Geometry check sheet. Reference: the model listing, model coordinates, mm. A direction names the side the tool comes from. Give positions to 0.01 mm unless a question says otherwise; leave off trailing zeros. Order: outer loops, then holes, each group sorted by start corner. A loop starts at its lowest first (then second) coordinate and runs counter-clockwise, first axis right, second up.
from build123d import *

# Parameters (mm, degrees)
SKETCH1_W           = 75
SKETCH1_H           = 15
BOSS_EXTRUDE1_DEPTH = 15
BOSS_EXTRUDE2_DEPTH = 7.5


with BuildPart() as part:
    # Sketch1 → Boss-Extrude1 (new, symmetric)
    with BuildSketch(Plane(origin=(0, 0, 0), x_dir=(-1, 0, 0), z_dir=(0, 1, 0))):
        with Locations((0, 7.5)):
            Rectangle(SKETCH1_W, SKETCH1_H)
    extrude(amount=BOSS_EXTRUDE1_DEPTH, both=True)

    # Sketch1_3 → Boss-Extrude2 (add, symmetric)
    with BuildSketch(Plane(origin=(0, 0, 0), x_dir=(-1, 0, 0), z_dir=(0, 1, 0))):
        Polygon((-22.5, 90), (-22.5, 15), (22.5, 15), (22.5, 90), (0, 112.5), align=None)
    extrude(amount=BOSS_EXTRUDE2_DEPTH, both=True)


solid = part.part
Item 1: Set-up check for faces 1 (the flat face through (0, -7.5, 64)), 2 (the flat face through (0, 7.5, 64)), 3 (the flat face through (-22.5, 0, 52)), 4 (the flat face through (22.5, 0, 53)), 5 (the flat face through (1, 0, 0)): record each of +Z, -Z, +X, -X, +Y, -Y from which the full face is reachable in a straight line by a thin tool's end or side.
Reported:
face 1: +Z, +X, -X, -Y
face 2: +Z, +X, -X, +Y
face 3: +Z, -X, +Y, -Y
face 4: +Z, +X, +Y, -Y
face 5: -Z, +X, -X, +Y, -Y
Item 2: Sectioned sample at B-B (y = -4.25). Enter the section's corners in (x, z).
Reported:
outline: (-37.5, 0) - (37.5, 0) - (37.5, 15) - (22.5, 15) - (22.5, 90) - (0, 112.5) - (-22.5, 90) - (-22.5, 15) - (-37.5, 15) - close
Item 3: Sectioned sample at A-A (x = -18.5). Enter the section's corners in (y, z), and give its area (4 significant figures).
Reported:
outline: (-15, 0) - (15, 0) - (15, 15) - (7.5, 15) - (7.5, 94) - (-7.5, 94) - (-7.5, 15) - (-15, 15) - close
area: 1,635 mm2
Item 4: Sectioned sample at D-D (x = -6). Enter the section's corners in (y, z).
Reported:
outline: (-15, 0) - (15, 0) - (15, 15) - (7.5, 15) - (7.5, 106.5) - (-7.5, 106.5) - (-7.5, 15) - (-15, 15) - close
Item 5: Scan lines: L1, parallel to Z at x = -16, y = 8.5; L2, parallel to X at y = -6.5, z = 83; L3, parallel to Y at x = -11.5, z = 41. Record each from-to range of solid material in increasing order.
Reported:
L1: z = 0 to 15
L2: x = -22.5 to 22.5
L3: y = -7.5 to 7.5
Item 6: Gauge pin test, flat ends, axial feed: pin 1 (4 mm diameter, centred on x = -4.5, z = 36, fed in from -Y); pin 2 (4.5 mm diameter, centred on y = 1, z = 58.5, fed in from -X); pin 3 (8 mm diameter, centred on x = 26, z = 66.5, fed in from +Y); pin 4 (1.5 mm diameter, centred on x = -8, y = 2.5, fed in from -Z). Record the tip position at first contact, or that the pin passes through.
Reported:
pin 1: stops at y = -7.5
pin 2: stops at x = -22.5
pin 3: stops at y = 7.5
pin 4: stops at z = 0
Item 7: Sectioned sample at C-C (z = 98). Enter the section's corners in (x, y), and give its area (3 significant figures).
Reported:
outline: (-14.5, -7.5) - (14.5, -7.5) - (14.5, 7.5) - (-14.5, 7.5) - close
area: 435 mm2
